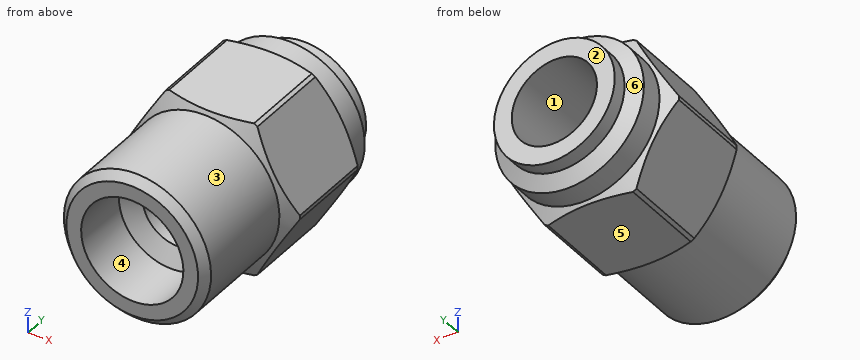
```python
from build123d import *

# Parameters (mm, degrees)
CUT_EXTRUDE1_DEPTH = 19.363823131
CHAMFER1_SIZE      = 0.5


with BuildPart() as part:
    # Sketch1 → Revolve1 (revolve)
    with BuildSketch(Plane(origin=(0, 0, 0), x_dir=(0, 0, -1), z_dir=(1, 0, 0)), mode=Mode.PRIVATE) as revolve1_sk:
        Polygon((4.75, 0), (4.75, 7), (5.7, 7.548482756), (5.7, 13.048482756), (4.8, 13.568097998), (4.8, 15.048482756), (3.9, 15.568097998), (3.9, 16.5), (2.75, 16.5), (2.75, 10.298482756), (2.2, 9.980940108), (2.2, 4.235085296), (3.3, 3.6), (3.3, 0), align=None)
    revolve(revolve1_sk.sketch.rotate(Axis((0, 19.630565864, 0), (0, -1, 0)), 180), axis=Axis((0, 19.630565864, 0), (0, -1, 0)))

    # Sketch2 → Cut-Extrude1 (cut, through all)
    with BuildSketch(Plane(origin=(0, 16.5, 0), x_dir=(1, 0, 0), z_dir=(0, 1, 0))):
        with BuildLine():
            Line((-2.886751346, 5), (2.886751346, 5))
            ThreePointArc((2.886751346, 5), (0, 5.773502692), (-2.886751346, 5))
        make_face()
        with BuildLine():
            Line((-5.773502692, 0), (-2.886751346, 5))
            ThreePointArc((-2.886751346, 5), (-5, 2.886751346), (-5.773502692, 0))
        make_face()
        with BuildLine():
            Line((-2.886751346, -5), (-5.773502692, 0))
            ThreePointArc((-5.773502692, 0), (-5, -2.886751346), (-2.886751346, -5))
        make_face()
        with BuildLine():
            ThreePointArc((-2.886751346, -5), (0, -5.773502692), (2.886751346, -5))
            Line((2.886751346, -5), (-2.886751346, -5))
        make_face()
        with BuildLine():
            ThreePointArc((2.886751346, -5), (5, -2.886751346), (5.773502692, 0))
            Line((5.773502692, 0), (2.886751346, -5))
        make_face()
        with BuildLine():
            ThreePointArc((5.773502692, 0), (5, 2.886751346), (2.886751346, 5))
            Line((2.886751346, 5), (5.773502692, 0))
        make_face()
    extrude(amount=-CUT_EXTRUDE1_DEPTH, mode=Mode.SUBTRACT)

    # Chamfer1
    chamfer1_edges = [part.edges().sort_by_distance(p)[0] for p in [
        (0, 0, -4.75),
    ]]
    chamfer(chamfer1_edges, length=CHAMFER1_SIZE)


solid = part.part
```
The listing builds one solid part. Answer for the finished solid, in the listing's coordinates (mm). Face numbers are marked on the shaded views. A direction names the side the tool comes from. Round coordinates to 2 decimals unless told otherwise and drop trailing zeros. Loops run counter-clockwise (first coordinate to the right, second up) from the corner with the lowest first, then second, coordinate; pieces in that order, holes last.
Q1. Section A-A, the plane y = 11.75 is taken. Determine the outline of the cut face in (x, z).
Q2. For a pull along Z with two mould halves and no side action, classify the marked faces 4, 5 and 6 as released by +Z, released by -Z, zero draft, split by the parting line, or undercut.
Q3. Find the intervals of material crossed by line 1 (X direction, y = 2.25, z = 0); line 2 (X direction, y = 3.75, z = -1.5); line 3 (Z direction, x = 0.75, y = 15.25), in increasing order.
Q4. Given pin 1 Ø3.5 at (x, z) = (0, 0) entering from +Y; pin 2 Ø5 at (x, y) = (1, 2) entering from -Z; pin 3 Ø1 at (y, z) = (7, -2) entering from +X; pin 4 Ø4 at (x, z) = (-0.5, 3) entering from -Y, each flat-ended and moving along its own axis, determine where each tip first touches the part or whether it passes through.
Q5. Which of the six approach directions +Z, -Z, +X, -X, +Y, -Y give full straight-line access (tool end or side, diameter ignored) to the marked faces 1, 2 and 3?
Completed:
1. outline: (-5.7, -0.13) - (-2.96, -4.87) arc R5.7 ccw to (-2.74, -5) - (2.74, -5) arc R5.7 ccw to (2.96, -4.87) - (5.7, -0.13) arc R5.7 ccw to (5.7, 0.13) - (2.96, 4.87) arc R5.7 ccw to (2.74, 5) - (-2.74, 5) arc R5.7 ccw to (-2.96, 4.87) - (-5.7, 0.13) arc R5.7 ccw to start; hole circle Ø5.5 at (0, 0)
2. face 4: undercut
2. face 5: released by -Z
2. face 6: split by the parting line
3. line 1: x = -4.75 to -3.3, 3.3 to 4.75
3. line 2: x = -4.51 to -2.64, 2.64 to 4.51
3. line 3: z = -4.39 to -2.65, 2.65 to 4.39
4. pin 1: passes through
4. pin 2: stops at z = -4.75
4. pin 3: stops at x = 4.88
4. pin 4: stops at y = 0
5. face 1: +Y
5. face 2: +Z, -Z, +X, -X, +Y
5. face 3: -Y
